Build history of the part. All positions in model axes, mm. A direction names the side the tool comes from. Coordinates: 2 decimals unless noted, no trailing zeros. Loops run counter-clockwise (first coordinate to the right, second up) from the corner with the lowest first, then second, coordinate; pieces in that order, holes last. Notation, with made-up numbers: (-40, -24.5) -> (9, -24.5) arc R23 ccw to (9, 4.5) -> close; hole circle Ø4 at (56.25, 87). An arc over 180 degrees is marked (long way). One line per item, written item: value. Start each with the question number.
```python
from build123d import *

# Parameters (mm, degrees)
PAD_DEPTH            = 11
POCKET_DEPTH         = 5.001
POCKET_DEPTH_BACK    = 5.001
POCKET001_DEPTH      = 11.314708
POCKET001_DEPTH_BACK = 11.314708
POCKET002_DEPTH      = 12.027279
POCKET002_DEPTH_BACK = 12.027279
FILLET_R             = 1


with BuildPart() as part:
    # Sketch → Pad (new body, symmetric)
    with BuildSketch(Plane.XZ):
        with BuildLine():
            Line((5, 5), (5, -7))
            Line((5, -7), (-5, -7))
            Line((-5, -7), (-5, 5))
            Line((-5, 5), (-2.897576, 5))
            ThreePointArc((-2.1, 4.262231), (-2.354338, 4.787276), (-2.897576, 5))
            Line((-2.1, 4.262231), (-1.862424, 1.217394))
            ThreePointArc((-1.926207, 0.836497), (-1.870986, 1.023039), (-1.862424, 1.217394))
            ThreePointArc((-1.926207, 0.836497), (0, -2.1), (1.926207, 0.836497))
            ThreePointArc((1.862424, 1.217394), (1.870986, 1.023039), (1.926207, 0.836497))
            Line((2.1, 4.262231), (1.862424, 1.217394))
            ThreePointArc((2.897576, 5), (2.354338, 4.787276), (2.1, 4.262231))
            Line((2.897576, 5), (5, 5))
        make_face()
    extrude(amount=PAD_DEPTH, both=True)

    # Sketch001 → Pocket (cut, two sides)
    with BuildSketch(Plane.YZ) as pocket_sk:
        Polygon((-0.3, -3.1), (0.3, -3.1), (0.3, 3.5), (0.5, 5), (-0.5, 5), (-0.3, 3.5), align=None)
    extrude(amount=-POCKET_DEPTH, mode=Mode.SUBTRACT)
    extrude(pocket_sk.sketch, amount=POCKET_DEPTH_BACK, mode=Mode.SUBTRACT)

    # Sketch002 → Pocket001 (cut, two sides)
    with BuildSketch(Plane(origin=(0, 0, 0), x_dir=(0.707107, 0.707107, 0), z_dir=(0.707107, -0.707107, 0))) as pocket001_sk:
        Polygon((-0.3, -3.1), (0.3, -3.1), (0.3, 3.5), (0.5, 5), (-0.5, 5), (-0.3, 3.5), align=None)
    extrude(amount=-POCKET001_DEPTH, mode=Mode.SUBTRACT)
    extrude(pocket001_sk.sketch, amount=POCKET001_DEPTH_BACK, mode=Mode.SUBTRACT)

    # Sketch003 → Pocket002 (cut, two sides)
    with BuildSketch(Plane(origin=(0, 0, 0), x_dir=(-0.866025, 0.5, 0), z_dir=(0.5, 0.866025, 0))) as pocket002_sk:
        Polygon((-0.3, -3.1), (0.3, -3.1), (0.3, 3.5), (0.5, 5), (-0.5, 5), (-0.3, 3.5), align=None)
    extrude(amount=-POCKET002_DEPTH, mode=Mode.SUBTRACT)
    extrude(pocket002_sk.sketch, amount=POCKET002_DEPTH_BACK, mode=Mode.SUBTRACT)

    # Fillet
    fillet_edges = [part.edges().sort_by_distance(p)[0] for p in [
        (-5, -11, -1),
        (-3.948788, -11, 5),
        (-5, -10.330127, 5),
        (-5, -4.080127, 5),
        (-5, 2.396447, 5),
        (-5, 8.353553, 5),
        (-5, 11, -1),
        (-3.948788, 11, 5),
        (5, 10.330127, 5),
        (5, 4.080127, 5),
        (5, 11, -1),
        (5, -11, -1),
        (5, -8.353553, 5),
        (5, -2.396447, 5),
    ]]
    fillet(fillet_edges, radius=FILLET_R)


solid = part.part
```
Item 1: Probe probe 1 along Y at (x, z) = (2.75, -1.25); probe 2 along X at (y, z) = (4.75, 4); probe 3 along Y at (x, z) = (-3.75, 0.25). List the from-to ranges inside material, lowest first.
Item 2: Drop a flat-ended pin along its axis: pin 1 Ø5.5 at (x, z) = (0, 0) entering from -Y. Give the stop position or say it passes through.
Item 3: Tool access for faces 4 (the face through (-2.279, -10.715, 2.695)), 5 (the face through (2.04, -0.87, -0.49)), 6 (the face through (-3, -0.3, 0)), 7 (the face through (3.046, -3.47, 0.246)): list every direction of +Z, -Z, +X, -X, +Y, -Y with a clear straight run to the whole face (end or side of a thin tool).
Item 4: Band-saw the part on B-B, the plane z = 0. Count the separate pieces of the cut face and the enclosed holes in it, and give its area (3 significant figures).
Item 5: Band-saw the part on A-A, the plane y = -7. List the corners of the cut face in (x, z), and give its area (3 significant figures).
Item 6: Two-plate mould, pull along X, no slides. Class faces 1 (the face through (-4.715, 7.391, 4.699)), 2 (the face through (3.573, 5.385, 4.261)), 3 (the face through (-3, 0.3, 0)): +X half, -X half, draft (parallel to the pull), parting line (faces both ways), or undercut.
Worked out:
1. probe 1: y = -11 to -3.17, -2.33 to -0.3, 0.3 to 4.16, 5.36 to 11
1. probe 2: x = -4.23 to -2.08, 2.08 to 2.32, 3.17 to 5
1. probe 3: y = -11 to -7.1, -5.9 to -0.3, 0.3 to 3.33, 4.17 to 11
2. pin 1: stops at y = -10.94
3. face 4: +Z, -Y
3. face 5: +Y, -Y
3. face 6: +Z, +X, -X
3. face 7: +Z
4. separate pieces: 8
4. enclosed holes: 0
4. area: 111 mm²
5. outline: (-5, -7) -> (5, -7) -> (5, 4) arc R1 ccw to (4, 5) -> (2.9, 5) arc R0.8 ccw to (2.1, 4.26) -> (1.86, 1.22) arc R0.8 ccw to (1.93, 0.84) arc R2.1 cw (long way) to (-1.93, 0.84) arc R0.8 ccw to (-1.86, 1.22) -> (-2.1, 4.26) arc R0.8 ccw to (-2.9, 5) -> (-3.46, 5) -> (-3.7, 3.5) -> (-3.7, -3.1) -> (-4.39, -3.1) -> (-4.39, 3.5) -> (-4.59, 4.81) arc R1 ccw to (-5, 4) -> close
5. area: 86.4 mm²
6. face 1: -X half
6. face 2: undercut
6. face 3: draft
